Geometry check sheet. Reference: drawing and pictorial views, mm from the part's lowest x, y, z. A direction names the side the tool comes from. Round coordinates to 2 decimals unless told otherwise and drop trailing zeros. Order: outer loops, then holes, each group sorted by start corner. A loop starts at its lowest first (then second) coordinate and runs counter-clockwise, first axis right, second up.
Q1. Mould release check, pull along Z, two halves, no side actions. Record for the marked faces 1, 2 and 3: +Z half, -Z half, draft (parallel to the pull), parting line (faces both ways), or undercut.
Q2. Scan lines: probe 1 along Z at (x, y) = (30, 23.75); probe 2 along Y at (x, z) = (30, 5.5); probe 3 along Z at (x, y) = (50, 22.25). Record each from-to range of solid material in increasing order.
Q3. Cross-section at C-C on z = 10. Record the cut outline in (x, y).
Q4. Cross-section at A-A on z = 30. Record the cut outline in (x, y), then the cut area to 3 significant figures.
Q5. Cross-section at B-B on x = 30. Record the cut outline in (y, z).
Q6. Depth check by flat-ended pin: P1, Ø1, axis at x = 30, z = 52, coming from the -Y side; P2, Ø9, axis at x = 30, z = 30, coming from the +Y side; P3, Ø5, axis at x = 41, y = 16, coming from the +Z side; P4, Ø5, axis at x = 12.5, y = 18.5, coming from the -Z side. Enter the tip coordinate at first touch or a pass-through.
Q7. Set-up check for the marked faces 4 and 5: record each of +Z, -Z, +X, -X, +Y, -Y from which the full face is reachable in a straight line by a thin tool's end or side.
Q8. Cross-section at D-D on x = 50. Record the cut outline in (y, z), then the cut area to 3 significant figures.
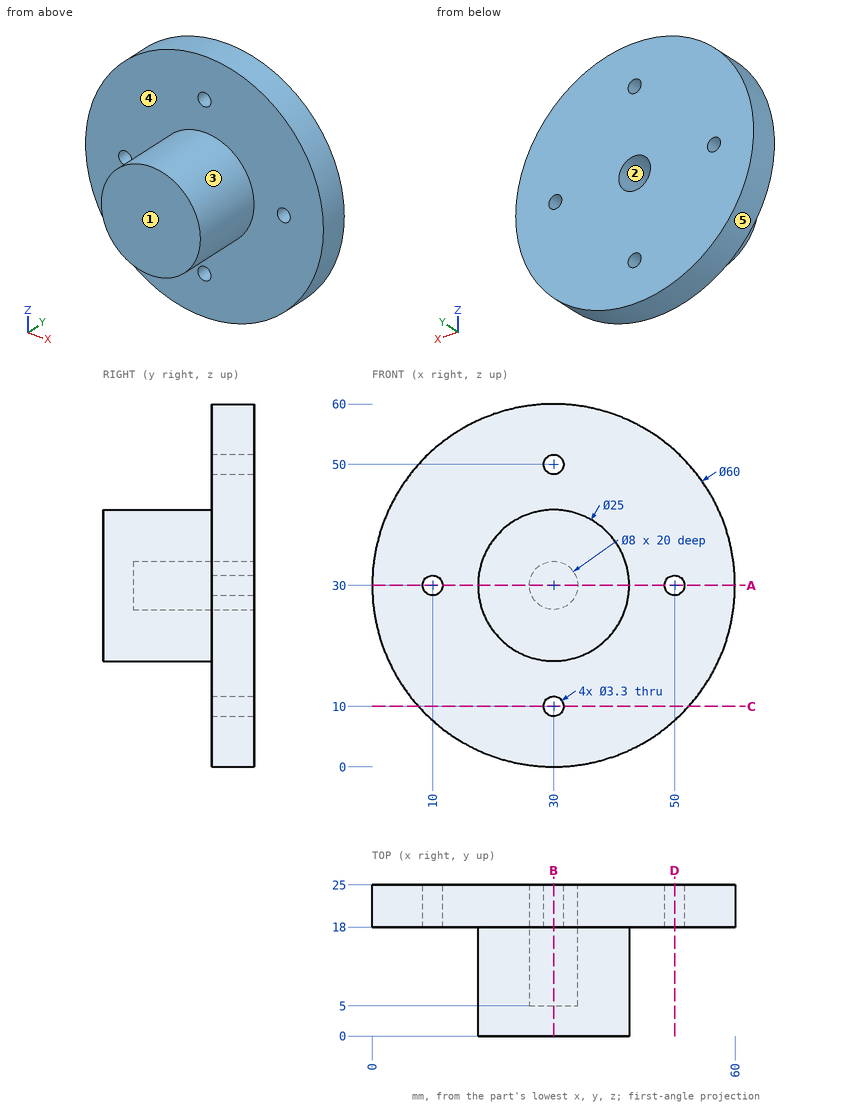
Results found:
1. face 1: draft
1. face 2: undercut
1. face 3: parting line
2. probe 1: z = 0 to 8.35, 11.65 to 26, 34 to 48.35, 51.65 to 60
2. probe 2: y = 18 to 25
2. probe 3: z = 7.64 to 28.35, 31.65 to 52.36
3. outline: (7.64, 18) - (28.35, 18) - (28.35, 25) - (7.64, 25) - close; (31.65, 18) - (52.36, 18) - (52.36, 25) - (31.65, 25) - close
4. outline: (0, 18) - (8.35, 18) - (8.35, 25) - (0, 25) - close; (11.65, 18) - (17.5, 18) - (17.5, 0) - (42.5, 0) - (42.5, 18) - (48.35, 18) - (48.35, 25) - (34, 25) - (34, 5) - (26, 5) - (26, 25) - (11.65, 25) - close; (51.65, 18) - (60, 18) - (60, 25) - (51.65, 25) - close
4. area: 664 mm2
5. outline: (0, 17.5) - (18, 17.5) - (18, 11.65) - (25, 11.65) - (25, 26) - (5, 26) - (5, 34) - (25, 34) - (25, 48.35) - (18, 48.35) - (18, 42.5) - (0, 42.5) - close; (18, 0) - (25, 0) - (25, 8.35) - (18, 8.35) - close; (18, 51.65) - (25, 51.65) - (25, 60) - (18, 60) - close
6. P1: stops at y = 18
6. P2: stops at y = 25
6. P3: stops at z = 58.46
6. P4: stops at z = 4.02
7. face 4: -Y
7. face 5: +Y, -Y
8. outline: (18, 7.64) - (25, 7.64) - (25, 28.35) - (18, 28.35) - close; (18, 31.65) - (25, 31.65) - (25, 52.36) - (18, 52.36) - close
8. area: 290 mm2
